Verification items for the finished model (mm, model axes). A direction names the side the tool comes from. Coordinates: 2 decimals unless noted, no trailing zeros. Loops run counter-clockwise (first coordinate to the right, second up) from the corner with the lowest first, then second, coordinate; pieces in that order, holes last. Notation, with made-up numbers: (40.25, 28.5) -> (58.25, 28.5) arc R6 cw to (58.25, 35.5) -> close; hole circle Ø1 at (23, 6). An arc over 180 degrees is marked (long way). Write item = value, one per line.
```python
from build123d import *

# Parameters (mm, degrees)
ESBO_O1_W                  = 120
ESBO_O1_H                  = 100
RESSALTO_EXTRUS_O1_DEPTH   = 4
ESBO_O2_W                  = 4
ESBO_O2_H                  = 4
ESBO_O2_W_2                = 112
ESBO_O2_H_2                = 92
RESSALTO_EXTRUS_O2_DEPTH   = 60
CORTE_EXTRUS_O1_DEPTH      = 26
CORTE_EXTRUS_O1_DEPTH_BACK = 23
FILETE1_R                  = 10
FILETE2_R                  = 10
FILETE3_R                  = 10
CORTE_EXTRUS_O2_DEPTH      = 37
CORTE_EXTRUS_O2_DEPTH_BACK = 36
F_3DSKETCH3_R              = 5.1
F_3DSKETCH3_R_2            = 3
CORTE_EXTRUS_O3_DEPTH      = 28
CORTE_EXTRUS_O3_DEPTH_BACK = 18


with BuildPart() as part:
    # Esboço1 → Ressalto-extrusão1 (new body)
    with BuildSketch(Plane.XY):
        with Locations((60, 50)):
            Rectangle(ESBO_O1_W, ESBO_O1_H)
    extrude(amount=RESSALTO_EXTRUS_O1_DEPTH)

    # Esboço2 → Ressalto-extrusão2 (add)
    with BuildSketch(Plane.XY):
        with Locations((2, 98)):
            Rectangle(ESBO_O2_W, ESBO_O2_H)
        with Locations((118, 98)):
            Rectangle(ESBO_O2_W, ESBO_O2_H)
        with Locations((60, 98)):
            Rectangle(ESBO_O2_W_2, ESBO_O2_H)
        with Locations((118, 50)):
            Rectangle(ESBO_O2_W, ESBO_O2_H_2)
        with Locations((118, 2)):
            Rectangle(ESBO_O2_W, ESBO_O2_H)
        with Locations((60, 2)):
            Rectangle(ESBO_O2_W_2, ESBO_O2_H)
        with Locations((2, 2)):
            Rectangle(ESBO_O2_W, ESBO_O2_H)
        with Locations((2, 50)):
            Rectangle(ESBO_O2_W, ESBO_O2_H_2)
    extrude(amount=RESSALTO_EXTRUS_O2_DEPTH)

    # 3DSketch1 → Corte-extrusão1 (cut, two sides)
    with BuildSketch(Plane(origin=(120, 14.15, 17.5), x_dir=(0, 0.9442477948596217, 0.32923563279624185), z_dir=(1, 0, 0))) as corte_extrus_o1_sk:
        Polygon((0, 0), (8.23089082, 23.606194871), (75.933457711, 0), (67.702566891, -23.606194871), align=None)
    extrude(amount=CORTE_EXTRUS_O1_DEPTH, mode=Mode.SUBTRACT)
    extrude(corte_extrus_o1_sk.sketch, amount=-CORTE_EXTRUS_O1_DEPTH_BACK, mode=Mode.SUBTRACT)

    # Filete1
    filete1_edges = [part.edges().sort_by_distance(p)[0] for p in [
        (120, 50, 0),
    ]]
    fillet(filete1_edges, radius=FILETE1_R)

    # Filete2
    filete2_edges = [part.edges().sort_by_distance(p)[0] for p in [
        (55, 0, 0),
        (120, 0, 35),
        (117.071067812, 0, 2.928932188),
    ]]
    fillet(filete2_edges, radius=FILETE2_R)

    # Filete3
    filete3_edges = [part.edges().sort_by_distance(p)[0] for p in [
        (120, 100, 35),
        (55, 100, 0),
        (117.071067812, 100, 2.928932188),
    ]]
    fillet(filete3_edges, radius=FILETE3_R)

    # 3DSketch2 → Corte-extrusão2 (cut, two sides)
    with BuildSketch(Plane(origin=(0, 83.957923226, 60), x_dir=(0, -0.8401982536854657, -0.5422793509842448), z_dir=(1, 0, 0))) as corte_extrus_o2_sk:
        Polygon((0, 0), (6.507352212, 10.082379044), (14.573255447, 4.876497275), (8.065903235, -5.205881769), align=None)
        Polygon((21.042782001, 0.700946272), (23.320355275, 4.229778938), (29.873901653, 0), (27.596328379, -3.528832665), align=None)
    extrude(amount=CORTE_EXTRUS_O2_DEPTH, mode=Mode.SUBTRACT)
    extrude(corte_extrus_o2_sk.sketch, amount=-CORTE_EXTRUS_O2_DEPTH_BACK, mode=Mode.SUBTRACT)

    # 3DSketch3 → Corte-extrusão3 (cut, two sides)
    with BuildSketch(Plane(origin=(0, 40.094193259, 48), x_dir=(0, -1, 0), z_dir=(-1, 0, 0))) as corte_extrus_o3_sk:
        with Locations(Location((0, 0, 0), (0, 0, 180))):
            Circle(F_3DSKETCH3_R)
        with Locations(Location((19.533873925, 0, 0), (0, 0, 180))):
            Circle(F_3DSKETCH3_R_2)
    extrude(amount=CORTE_EXTRUS_O3_DEPTH, mode=Mode.SUBTRACT)
    extrude(corte_extrus_o3_sk.sketch, amount=-CORTE_EXTRUS_O3_DEPTH_BACK, mode=Mode.SUBTRACT)


solid = part.part
```
1) Release check for a two-part mould opening along X. For faces 1 (the face through (2, 83.958, 54)), 2 (the face through (4, 49, 32)), 3 (the face through (116.99, 2.85, 35.35)) record: pulls with the +X half, pulls with the -X half, needs draft (parallel to the pull), parting line crosses it, or undercut.
Ans:
face_1 = needs draft
face_2 = undercut
face_3 = pulls with the +X half
2) Material ranges on line 1 (Y direction, x = 55.5, z = 11); line 2 (X direction, y = 14, z = 32.5); line 3 (X direction, y = 64.5, z = 21.5), recorded low to high.
Ans:
line_1 = 0 to 4, 96 to 100
line_2 = 0 to 4, 116 to 120
line_3 = 0 to 4
3) Depth check by flat-ended pin: pin 1 Ø1 at (x, y) = (12.5, 63) entering from +Z; pin 2 Ø1.2 at (x, z) = (117.5, 26) entering from +Y; pin 3 Ø1.2 at (x, z) = (117.5, 32.5) entering from -Y. Enter the tip coordinate at first touch or a pass-through.
Ans:
pin_1 = 4
pin_2 = 97.24
pin_3 = 2.76
4) Sectioned sample at B-B, the plane z = 41. Record the cut outline in (x, y).
Ans:
outline = (0, 0) -> (110, 0) arc R10 ccw to (120, 10) -> (120, 14.15) -> (116, 14.15) -> (116, 4) -> (4, 4) -> (4, 96) -> (116, 96) -> (116, 85.85) -> (120, 85.85) -> (120, 90) arc R10 ccw to (110, 100) -> (0, 100) -> close
5) Sectioned sample at A-A, the plane y = 57. Record the cut outline in (x, z), plus the area to 3 significant figures.
Ans:
outline = (0, 0) -> (110, 0) arc R10 ccw to (120, 10) -> (120, 17.5) -> (116, 17.5) -> (116, 4) -> (4, 4) -> (4, 60) -> (0, 60) -> close; (116, 42.5) -> (120, 42.5) -> (120, 60) -> (116, 60) -> close
area = 807 mm2
6) Sectioned sample at D-D, the plane z = 56.5. Record the cut outline in (x, y), plus the area to 3 significant figures.
Ans:
outline = (0, 0) -> (110, 0) arc R10 ccw to (120, 10) -> (120, 90) arc R10 ccw to (110, 100) -> (0, 100) -> (0, 83.96) -> (4, 83.96) -> (4, 96) -> (116, 96) -> (116, 4) -> (4, 4) -> (4, 74.36) -> (0, 74.36) -> close
area = 1,610 mm2
7) Tool access check on faces 4 (the face through (2, 35, 47.8)), 5 (the face through (2, 79, 48)), 6 (the face through (118, 51, 17.5)), 7 (the face through (59, 96, 32)), 8 (the face through (117.15, 96.99, 34.65)). Record the directions out of +Z, -Z, +X, -X, +Y, -Y that give a thin tool (end or side, any length) a straight path to the whole face; none if there is none.
Ans:
face_4 = -X
face_5 = +Z, -X
face_6 = +X
face_7 = +Z
face_8 = +Z, -Z, +X, +Y
8) Sectioned sample at C-C, the plane x = 90.5. Record the cut outline in (y, z), plus the area to 3 significant figures.
Ans:
outline = (0, 10) arc R10 ccw to (10, 0) -> (90, 0) arc R10 ccw to (100, 10) -> (100, 60) -> (96, 60) -> (96, 4) -> (4, 4) -> (4, 60) -> (0, 60) -> close
area = 805 mm2
